from build123d import *

# Parameters (mm, degrees)
BOSS_EXTRUDE1_DEPTH = 11.5
SKETCH2_R           = 2.65
CUT_EXTRUDE1_DEPTH  = 30.533878851
SKETCH3_R           = 2.65
CUT_EXTRUDE2_DEPTH  = 30.533878851


with BuildPart() as part:
    # Sketch1 → Boss-Extrude1 (new body)
    with BuildSketch(Plane(origin=(0, 0, 0), x_dir=(0, 0, -1), z_dir=(1, 0, 0))):
        Polygon((0, 0), (22, 0), (22, 22), (16, 22), (16, 6), (0, 6), align=None)
    extrude(amount=-BOSS_EXTRUDE1_DEPTH)

    # Sketch2 → Cut-Extrude1 (cut, through all)
    with BuildSketch(Plane(origin=(0, 6, 0), x_dir=(1, 0, 0), z_dir=(0, 1, 0))):
        with Locations(Location((-5.75, 8, 0), (0, 0, 270))):
            Circle(SKETCH2_R)
    extrude(amount=-CUT_EXTRUDE1_DEPTH, mode=Mode.SUBTRACT)

    # Sketch3 → Cut-Extrude2 (cut, through all)
    with BuildSketch(Plane.XY.offset(-16)):
        with Locations((-5.75, 14)):
            Circle(SKETCH3_R)
    extrude(amount=-CUT_EXTRUDE2_DEPTH, mode=Mode.SUBTRACT)


solid = part.part
Check sheet for the modelled part. Datum: model origin and axes. Units: mm. A direction names the side the tool comes from. Give positions to 0.01 mm unless a question says otherwise; leave off trailing zeros. Write each loop counter-clockwise with the first axis right and the second up, starting at its lowest first coordinate (ties: lowest second). Pieces come first, ordered by that corner, then holes. Notation, with made-up numbers: (38.5, 70) -> (85.5, 70) arc R26 cw to (85.5, 95) -> close; hole circle Ø1 at (42.25, 84). An arc over 180 degrees is marked (long way). Use one line per item in the form item = value. Start each with the question number.
1. Mould release check, pull along Y, two halves, no side actions. Record for faces 1 (the cylindrical face through (-6.32, 11.41, -18.96)), 2 (the flat face through (-11.5, 4, -16)), 3 (the flat face through (-6, 22, -19)): pulls with the +Y half, pulls with the -Y half, needs draft (parallel to the pull), parting line crosses it, or undercut.
2. Section check A-A (y = 14). Record the cut outline in (x, z).
3. Go/stop test with a flat-tipped pin: P1, Ø3.5, axis at x = -7, z = -7, coming from the +Y side. Record where the tip stops, or that it passes through.
4. Thickness scan on line 1 along X through (y, z) = (4.2, -8); line 2 along Z through (x, y) = (-8, 10.25); line 3 along Y through (x, z) = (-5.75, -17.7). Record the ranges inside material, lowest first. Write a range as from..to.
5. Section check D-D (y = 4). Record the cut outline in (x, z).
6. Section check B-B (z = -8). Record the cut outline in (x, y).
7. Access from +Z, -Z, +X, -X, +Y, -Y to the whole of each face (thin tool, end or side, straight path). Record for faces 4 (the flat face through (-3, 16, -16)), 5 (the flat face through (-6, 3, 0)).
8. Section check C-C (x = -5.75). Record the cut outline in (y, z).
Conclusion:
q1.face_1 = undercut
q1.face_2 = needs draft
q1.face_3 = pulls with the +Y half
q2.outline = (-11.5, -22) -> (-8.4, -22) -> (-8.4, -16) -> (-11.5, -16) -> close; (-3.1, -22) -> (0, -22) -> (0, -16) -> (-3.1, -16) -> close
q3.P1 = 6
q4.line_1 = -11.5..-8.4, -3.1..0
q4.line_2 = -22..-16
q4.line_3 = 0..11.35, 16.65..22
q5.outline = (-11.5, -22) -> (0, -22) -> (0, 0) -> (-11.5, 0) -> close; hole circle Ø5.3 at (-5.75, -8)
q6.outline = (-11.5, 0) -> (-8.4, 0) -> (-8.4, 6) -> (-11.5, 6) -> close; (-3.1, 0) -> (0, 0) -> (0, 6) -> (-3.1, 6) -> close
q7.face_4 = +Z, +X, -X, +Y
q7.face_5 = +Z, +X, -X, +Y, -Y
q8.outline = (0, -22) -> (11.35, -22) -> (11.35, -16) -> (6, -16) -> (6, -10.65) -> (0, -10.65) -> close; (0, -5.35) -> (6, -5.35) -> (6, 0) -> (0, 0) -> close; (16.65, -22) -> (22, -22) -> (22, -16) -> (16.65, -16) -> close
